from build123d import *

# Parameters (mm, degrees)
SKETCH_1_W          = 4.5
SKETCH_1_H          = 12
EXTRUDE_1_DEPTH     = 2
EXTRUDE_1_2_DEPTH   = 2
SKETCH_2_W          = 4.5
SKETCH_2_H          = 12
EXTRUDE_4_DEPTH     = 2
SKETCH_4_R          = 1.5
CUT_EXTRUDE_1_DEPTH = 18.413285158
SKETCH_5_W          = 31.7
SKETCH_5_H          = 5.5
EXTRUDE_5_DEPTH     = 2
SKETCH_6_W          = 31.7
SKETCH_6_H          = 2
EXTRUDE_6_DEPTH     = 15
SKETCH_7_W          = 22.5
SKETCH_7_H          = 2
EXTRUDE_7_DEPTH     = 15.5
FILLET_3_R          = 1
FILLET_4_R          = 4.5
FILLET_5_R          = 1
FILLET_6_R          = 3
SKETCH_8_W          = 4.5
SKETCH_8_H          = 2
EXTRUDE_8_DEPTH     = 5.5
FILLET_7_R          = 2
CUT_EXTRUDE_2_DEPTH = 28.936938031
FILLET_8_R          = 0.5


with BuildPart() as part:
    # Sketch 1 → Extrude 1 (new body)
    with BuildSketch(Plane.XY):
        with Locations((13.6, 0)):
            Rectangle(SKETCH_1_W, SKETCH_1_H)
    extrude(amount=EXTRUDE_1_DEPTH)


with BuildPart() as body_2:
    # Sketch 1 → Extrude 1 2 (new body)
    with BuildSketch(Plane.XY):
        with Locations((-13.6, 0)):
            Rectangle(SKETCH_1_W, SKETCH_1_H)
    extrude(amount=EXTRUDE_1_2_DEPTH)

    # Sketch 2 → Extrude 4 (add)
    with BuildSketch(Plane.XY):
        with Locations((-13.6, 0)):
            Rectangle(SKETCH_2_W, SKETCH_2_H)
    extrude(amount=-EXTRUDE_4_DEPTH)


with BuildPart() as cut_extrude_1_tool:
    # Sketch 4 → Cut-Extrude 1 (new, through all)
    with BuildSketch(Plane(origin=(0, 0, 2), x_dir=(-1, 0, 0), z_dir=(0, 0, -1))):
        with Locations((13.6, 0)):
            Circle(SKETCH_4_R)
        with Locations(Location((-13.6, 0, 0), (0, 0, 180))):
            Circle(SKETCH_4_R)
    extrude(amount=CUT_EXTRUDE_1_DEPTH)


with BuildPart() as part_1:
    add(part.part)

    # Cut-Extrude 1: cut by cut_extrude_1_tool
    add(cut_extrude_1_tool.part, mode=Mode.SUBTRACT)



with BuildPart() as body_2_1:
    add(body_2.part)

    # Cut-Extrude 1: cut by cut_extrude_1_tool
    add(cut_extrude_1_tool.part, mode=Mode.SUBTRACT)


with BuildPart() as part_2:
    add(part_1.part)

    add(body_2_1.part)  # Extrude 5 merges body 2
    # Sketch 5 → Extrude 5 (add)
    with BuildSketch(Plane.XY.offset(2)):
        with Locations((0, 8.75)):
            Rectangle(SKETCH_5_W, SKETCH_5_H)
    extrude(amount=-EXTRUDE_5_DEPTH)

    # Sketch 6 → Extrude 6 (add)
    with BuildSketch(Plane.XY.offset(2)):
        with Locations((0, 10.5)):
            Rectangle(SKETCH_6_W, SKETCH_6_H)
    extrude(amount=EXTRUDE_6_DEPTH)

    # Sketch 7 → Extrude 7 (add)
    with BuildSketch(Plane.XZ.offset(-9.5)):
        with Locations((0, 16)):
            Rectangle(SKETCH_7_W, SKETCH_7_H)
    extrude(amount=EXTRUDE_7_DEPTH)

    # Fillet 3
    fillet_3_edges = [part_2.edges().sort_by_distance(p)[0] for p in [
        (-15.85, -6, 0),
        (15.85, -6, 1),
        (11.25, -6, 16),
        (-11.25, -6, 16),
    ]]
    fillet(fillet_3_edges, radius=FILLET_3_R)

    # Fillet 4
    fillet_4_edges = [part_2.edges().sort_by_distance(p)[0] for p in [
        (11.25, 9.5, 16),
        (-11.25, 9.5, 16),
    ]]
    fillet(fillet_4_edges, radius=FILLET_4_R)

    # Fillet 5
    fillet_5_edges = [part_2.edges().sort_by_distance(p)[0] for p in [
        (0, 9.5, 2),
        (0, 9.5, 15),
    ]]
    fillet(fillet_5_edges, radius=FILLET_5_R)

    # Fillet 6
    fillet_6_edges = [part_2.edges().sort_by_distance(p)[0] for p in [
        (15.85, 10.5, 17),
        (-15.85, 10.5, 17),
    ]]
    fillet(fillet_6_edges, radius=FILLET_6_R)

    # Sketch 8 → Extrude 8 (add)
    with BuildSketch(Plane(origin=(0, 6, 0), x_dir=(1, 0, 0), z_dir=(0, 1, 0))):
        with Locations((-13.6, 1)):
            Rectangle(SKETCH_8_W, SKETCH_8_H)
    extrude(amount=EXTRUDE_8_DEPTH)

    # Fillet 7
    fillet_7_edges = [part_2.edges().sort_by_distance(p)[0] for p in [
        (-11.35, 8.75, 0),
    ]]
    fillet(fillet_7_edges, radius=FILLET_7_R - 0.0001)  # a hair under: the kernel refuses the full size

    # Sketch 9 → Cut-Extrude 2 (cut, through all)
    with BuildSketch(Plane.XZ.offset(-9.5)):
        Polygon((-15.85, 9.25), (-13.85, 9.25), (-13.85, 10.5), (-12.35, 10.5), (-12.35, 6.5), (-13.85, 6.5), (-13.85, 7.75), (-15.85, 7.75), align=None)
    extrude(amount=-CUT_EXTRUDE_2_DEPTH, mode=Mode.SUBTRACT)

    # Fillet 8
    fillet_8_edges = [part_2.edges().sort_by_distance(p)[0] for p in [
        (-15.85, 10.5, 7.75),
        (-15.85, 10.5, 9.25),
        (-13.85, 10.5, 9.25),
        (-13.85, 10.5, 10.5),
        (-12.35, 10.5, 10.5),
        (-12.35, 10.5, 6.5),
        (-13.85, 10.5, 6.5),
        (-13.85, 10.5, 7.75),
    ]]
    fillet(fillet_8_edges, radius=FILLET_8_R)


solid = part_2.part
Can you work these out from the model? Positions are in its coordinate system, mm. A direction names the side the tool comes from. Round coordinates to 2 decimals unless told otherwise and drop trailing zeros. Loops run counter-clockwise (first coordinate to the right, second up) from the corner with the lowest first, then second, coordinate; pieces in that order, holes last. Notation, with made-up numbers: (86, 29.5) - (127, 29.5) arc R29 ccw to (127, 66.5) - close; hole circle Ø10 at (20.25, 79.5). An arc over 180 degrees is marked (long way). Answer in a Markdown table with one row per item. Add a question column.
Q1. I want a section at B-B on x = -0.5. List the corners of the cut face in (y, z) for me, and give its area (3 significant figures).
Q2. For pin 1 Ø4 at (x, y) = (13.6, 0) entering from -Z; pin 2 Ø0.8 at (x, y) = (-15, 10) entering from +Z; pin 3 Ø3 at (x, z) = (1.5, -0.5) entering from -Y, each with a flat end and sliding along its axis, tell me the tip position at first contact or that it passes through.
Q3. We'd pull the mould along Z, two halves only. Please class faces 5 (the flat face through (0, 9.5, 7)), 6 (the flat face through (-11.25, 0, 16)), 7 (the cylindrical face through (-10.78, 8.79, -0.6)): pulls with the +Z half, pulls with the -Z half, needs draft (parallel to the pull), parting line crosses it, or undercut.
Q4. I want a section at A-A on y = 0. List the corners of the cut face in (x, z) for me, and give its area (3 significant figures).
Q5. Which directions (+Z, -Z, +X, -X, +Y, -Y) give clear straight access to the entire face, cutting with the end or side of a thin tool? Please do faces 1 (the flat face through (0, 1, 15)), 2 (the cylindrical face through (-12.1, 0.07, 0.03)), 3 (the flat face through (-12.35, 10, 9)), 4 (the flat face through (6, 7, 0)).
Q6. I need wall thicknesses on L1, parallel to X at y = 0, z = -0.45; L2, parallel to Y at x = -13.6, z = 0.35; L3, parallel to Z at x = -2.5, y = 8.5. Which ranges of each line are inside material? Lowest first, please.
Q7. I want a section at C-C on x = 13.6. List the corners of the cut face in (y, z) for me, and give its area (3 significant figures).
A:
| question | item | result |
|---|---|---|
| 1 | outline | (-6, 15) - (8.5, 15) arc R1 cw to (9.5, 14) - (9.5, 3) arc R1 cw to (8.5, 2) - (6, 2) - (6, 0) - (11.5, 0) - (11.5, 17) - (-6, 17) - close |
| 1 | area | 72.4 mm^2 |
| 2 | pin 1 | z = 0 |
| 2 | pin 2 | z = 16.44 |
| 2 | pin 3 | y = 6 |
| 3 | face 5 | undercut |
| 3 | face 6 | needs draft |
| 3 | face 7 | pulls with the -Z half |
| 4 | outline | (-15.85, -2) - (-15.1, -2) - (-15.1, 2) - (-15.85, 2) - close; (-12.1, -2) - (-11.35, -2) - (-11.35, 2) - (-12.1, 2) - close; (-11.25, 15) - (11.25, 15) - (11.25, 17) - (-11.25, 17) - close; (11.35, 0) - (12.1, 0) - (12.1, 2) - (11.35, 2) - close; (15.1, 0) - (15.85, 0) - (15.85, 2) - (15.1, 2) - close |
| 4 | area | 54.0 mm^2 |
| 5 | face 1 | +X, -X, -Y |
| 5 | face 2 | +Z, -Z |
| 5 | face 3 | +Y, -Y |
| 5 | face 4 | -Z, +X, +Y, -Y |
| 6 | L1 | -15.85 to -15.1, -12.1 to -11.35 |
| 6 | L2 | -6 to -1.5, 1.5 to 11.5 |
| 6 | L3 | 0 to 2, 15 to 17 |
| 7 | outline | (-6, 0) - (-1.5, 0) - (-1.5, 2) - (-6, 2) - close; (1.5, 0) - (11.5, 0) - (11.5, 16.9) - (8.95, 16.9) - (8.95, 14.89) arc R1 cw to (9.5, 14) - (9.5, 3) arc R1 cw to (8.5, 2) - (1.5, 2) - close |
| 7 | area | 60.3 mm^2 |
